from build123d import *

# Parameters (mm, degrees)
F1_W     = 50.8
F1_H     = 50.8
F1_R     = 12.7
F2_DEPTH = 50.8
F3_W     = 30.162047
F3_H     = 25.4
F4_DEPTH = 12.7
F5_W     = 30.217611
F5_H     = 25.4
F6_DEPTH = 12.7


with BuildPart() as f2:
    # F1 (on face) → F2 (new body)
    with BuildSketch(Plane.XZ):
        with Locations((25.4, 25.4)):
            Rectangle(F1_W, F1_H)
        with Locations((24.368526, 27.008452)):
            Circle(F1_R, mode=Mode.SUBTRACT)
    extrude(amount=F2_DEPTH)

    # F3 (on face) → F4 (join)
    with BuildSketch(Plane(origin=(0, 0, 0), x_dir=(1, 0, 0), z_dir=(0, 0, -1))):
        with Locations((24.673132, 25.4)):
            Rectangle(F3_W, F3_H)
    extrude(amount=F4_DEPTH)

    # F5 (on face) → F6 (join)
    with BuildSketch(Plane.YZ.offset(50.8)):
        with Locations((-24.774669, 25.4)):
            Rectangle(F5_W, F5_H)
    extrude(amount=F6_DEPTH)


solid = f2.part
Work out the finished part from the listing and answer in its coordinate system (mm). A direction names the side the tool comes from. Coordinates: 2 decimals unless noted, no trailing zeros. Order: outer loops, then holes, each group sorted by start corner. A loop starts at its lowest first (then second) coordinate and runs counter-clockwise, first axis right, second up. Notation, with made-up numbers: (-4.5, 0) - (36.5, 0) arc R15 ccw to (36.5, 12) - close; hole circle Ø1 at (-34, -1.75). An arc over 180 degrees is marked (long way). Put each result on its own line as item: value. Start each with the question number.
1) Find section A-A (z = 26). Give the vertices of the cut face in (x, y).
2) Find the intervals of material crossed by line 1 (X direction, y = -2.5, z = 26.5); line 2 (Z direction, x = 53.5, y = -34.5); line 3 (Y direction, x = 60.5, z = 21), in increasing order. Write a range as from..to.
3) Flat-ended cylindrical pins translate along their axes: pin 1 (1 mm diameter, centred on x = 54, z = 23, fed in from -Y); pin 2 (4 mm diameter, centred on x = 28, z = -7, fed in from -Y); pin 3 (6.5 mm diameter, centred on x = 55.5, z = 22.5, fed in from +Y). Find the tip coordinate at first contact, or state that the pin passes through.
4) Find section D-D (z = 43). Give the vertices of the cut face in (x, y).
5) For faces 1 (the flat face through (9.592, -25, -6)), 2 (the flat face through (24, -38.1, -6)), 3 (the flat face through (24, -12.7, -6)), 4 (the flat face through (39.754, -25, -6)), determine the directions among +Z, -Z, +X, -X, +Y, -Y from which every point of the face is accessible in a straight line to the end or side of a thin tool.
6) For a pull along Z with two mould halves and no side action, classify faces 5 (the cylindrical face through (31.196, -25.044, 37.717)), 6 (the flat face through (57, -9.666, 25)), 7 (the flat face through (57, -25, 38.1)), 8 (the flat face through (57, -25, 12.7)) as released by +Z, released by -Z, zero draft, split by the parting line, or undercut.
7) Find section C-C (y = -7). Give the vertices of the cut face in (x, z).
8) Find section B-B (x = 24). Give the vertices of the cut face in (y, z), plus the area to 3 significant figures.
Results list:
1. outline: (0, -50.8) - (11.71, -50.8) - (11.71, 0) - (0, 0) - close; (37.03, -50.8) - (50.8, -50.8) - (50.8, -39.88) - (63.5, -39.88) - (63.5, -9.67) - (50.8, -9.67) - (50.8, 0) - (37.03, 0) - close
2. line 1: x = 0..11.68, 37.06..50.8
2. line 2: z = 12.7..38.1
2. line 3: y = -39.88..-9.67
3. pin 1: stops at y = -39.88
3. pin 2: stops at y = -38.1
3. pin 3: stops at y = -9.67
4. outline: (0, -50.8) - (50.8, -50.8) - (50.8, 0) - (0, 0) - close
5. face 1: -Z, -X, +Y, -Y
5. face 2: -Z, +X, -X, -Y
5. face 3: -Z, +X, -X, +Y
5. face 4: -Z, +X, +Y, -Y
6. face 5: undercut
6. face 6: zero draft
6. face 7: released by +Z
6. face 8: released by -Z
7. outline: (0, 0) - (50.8, 0) - (50.8, 50.8) - (0, 50.8) - close; hole circle Ø25.4 at (24.37, 27.01)
8. outline: (-50.8, 0) - (-38.1, 0) - (-38.1, -12.7) - (-12.7, -12.7) - (-12.7, 0) - (0, 0) - (0, 14.31) - (-50.8, 14.31) - close; (-50.8, 39.7) - (0, 39.7) - (0, 50.8) - (-50.8, 50.8) - close
8. area: 1,610 mm^2
